Input: part model. Units: mm. Frame: model coordinates. Face numbers are marked on the shaded views. A direction names the side the tool comes from. Give positions to 0.01 mm unless a question says otherwise; leave off trailing zeros. Loops run counter-clockwise (first coordinate to the right, second up) from the corner with the lowest first, then second, coordinate; pieces in that order, holes last. Notation, with made-up numbers: (-38.5, 64) -> (-12.5, 64) arc R28 cw to (-12.5, 91) -> close; hole circle Ø1 at (65, -2.75). An arc over 180 degrees is marked (long way). Answer in a Markdown table with one row per item. Add a question column.
```python
from build123d import *

# Parameters (mm, degrees)
SKETCH1_W           = 57
SKETCH1_H           = 37
BOSS_EXTRUDE1_DEPTH = 44
SKETCH2_W           = 38.4
SKETCH2_H           = 36
CUT_EXTRUDE1_DEPTH  = 47
BOSS_EXTRUDE2_DEPTH = 20
BOSS_EXTRUDE3_DEPTH = 20
SKETCH7_W           = 53
SKETCH7_H           = 31
CUT_EXTRUDE4_DEPTH  = 8
SKETCH8_R           = 1.9
CUT_EXTRUDE5_DEPTH  = 40
SKETCH10_W          = 57
SKETCH10_H          = 77
BOSS_EXTRUDE4_DEPTH = 10
SKETCH12_W          = 38.4
SKETCH12_H          = 77
CUT_EXTRUDE6_DEPTH  = 8


with BuildPart() as part:
    # Sketch1 → Boss-Extrude1 (new body)
    with BuildSketch(Plane(origin=(0, 0, 0), x_dir=(1, 0, 0), z_dir=(0, 1, 0))):
        Rectangle(SKETCH1_W, SKETCH1_H)
    extrude(amount=BOSS_EXTRUDE1_DEPTH)

    # Sketch2 → Cut-Extrude1 (cut)
    with BuildSketch(Plane.XY.offset(18.5)):
        with Locations((0, 18)):
            Rectangle(SKETCH2_W, SKETCH2_H)
    extrude(amount=-CUT_EXTRUDE1_DEPTH, mode=Mode.SUBTRACT)

    # Sketch5 → Boss-Extrude2 (add)
    with BuildSketch(Plane(origin=(0, 0, -18.5), x_dir=(-1, 0, 0), z_dir=(0, 0, -1))):
        Polygon((-19.2, 36), (19.2, 36), (19.2, 0), (28.5, 0), (28.5, 44), (-28.5, 44), (-28.5, 0), (-19.2, 0), align=None)
    extrude(amount=BOSS_EXTRUDE2_DEPTH)

    # Sketch6 → Boss-Extrude3 (add)
    with BuildSketch(Plane.XY.offset(18.5)):
        Polygon((-28.5, 0), (-19.2, 0), (-19.2, 36), (19.2, 36), (19.2, 0), (28.5, 0), (28.5, 44), (-28.5, 44), align=None)
    extrude(amount=BOSS_EXTRUDE3_DEPTH)

    # Sketch7 → Cut-Extrude4 (cut)
    with BuildSketch(Plane(origin=(0, 44, 0), x_dir=(1, 0, 0), z_dir=(0, 1, 0))):
        with Locations((-2, 0)):
            Rectangle(SKETCH7_W, SKETCH7_H)
    extrude(amount=-CUT_EXTRUDE4_DEPTH, mode=Mode.SUBTRACT)

    # Sketch8 → Cut-Extrude5 (cut)
    with BuildSketch(Plane(origin=(0, 44, 0), x_dir=(1, 0, 0), z_dir=(0, 1, 0))):
        with Locations(Location((23.85, -27, 0), (0, 0, 270))):
            Circle(SKETCH8_R)
        with Locations(Location((-23.85, -27, 0), (0, 0, 270))):
            Circle(SKETCH8_R)
        with Locations(Location((-23.85, 27, 0), (0, 0, 270))):
            Circle(SKETCH8_R)
        with Locations(Location((23.85, 27, 0), (0, 0, 270))):
            Circle(SKETCH8_R)
    extrude(amount=-CUT_EXTRUDE5_DEPTH, mode=Mode.SUBTRACT)

    # Sketch10 → Boss-Extrude4 (add)
    with BuildSketch(Plane.XZ):
        Rectangle(SKETCH10_W, SKETCH10_H)
    extrude(amount=BOSS_EXTRUDE4_DEPTH)

    # Sketch12 → Cut-Extrude6 (cut)
    with BuildSketch(Plane(origin=(0, 44, 0), x_dir=(1, 0, 0), z_dir=(0, 1, 0))):
        Rectangle(SKETCH12_W, SKETCH12_H)
    extrude(amount=-CUT_EXTRUDE6_DEPTH, mode=Mode.SUBTRACT)


solid = part.part
```
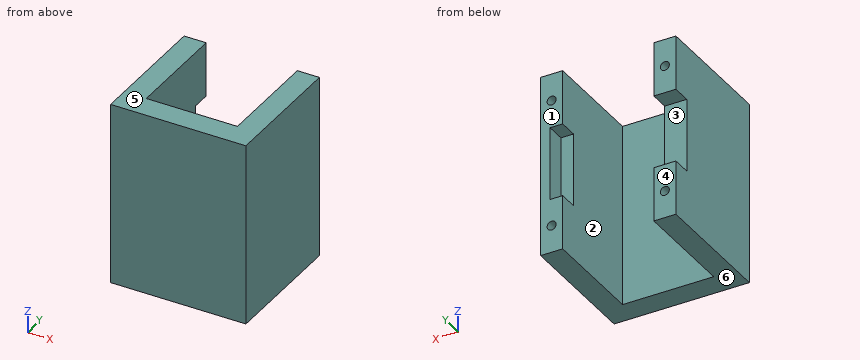
1) Section A-A on y = 6. Output: boundary loops of the cut face in (x, z), and give its area (3 significant figures).
2) Pin query (flat end, axial travel): pin 1 (4 mm diameter, centred on x = -7.5, z = -26.5, fed in from +Y); pin 2 (7.5 mm diameter, centred on x = -22, z = 4.5, fed in from +Y). Return the tip coordinate at first contact, or that it passes through.
3) Section C-C on x = -23.85. Output: boundary loops of the cut face in (y, z).
4) Section D-D on z = -27. Output: boundary loops of the cut face in (x, y).
5) Pull-direction query (Z, two-part tool) for the marked faces 3, 4, 5 and 6; classes: +Z half, -Z half, draft (parallel to the pull), parting line (faces both ways), or undercut.
6) Section B-B on z = 31. Output: boundary loops of the cut face in (x, y).
7) Material intervals for line 1 along X through (y, z) = (20, 27); line 2 along X through (y, z) = (14, -6); line 3 along Z through (x, y) = (-23, 23), sorted ascending.
8) Reachability of the marked faces 1 and 2 from +Z, -Z, +X, -X, +Y, -Y: full face, straight path, thin tool, end or side. Return the list, or none.
Working result:
| question | item | result |
|---|---|---|
| 1 | outline | (-28.5, -38.5) -> (-19.2, -38.5) -> (-19.2, 38.5) -> (-28.5, 38.5) -> close; (19.2, -38.5) -> (28.5, -38.5) -> (28.5, 38.5) -> (19.2, 38.5) -> close; hole circle Ø3.8 at (-23.85, -27); hole circle Ø3.8 at (-23.85, 27); hole circle Ø3.8 at (23.85, -27); hole circle Ø3.8 at (23.85, 27) |
| 1 | area | 1,390 mm2 |
| 2 | pin 1 | stops at y = 0 |
| 2 | pin 2 | stops at y = 36 |
| 3 | outline | (-10, -38.5) -> (44, -38.5) -> (44, -28.9) -> (4, -28.9) -> (4, -25.1) -> (44, -25.1) -> (44, -15.5) -> (36, -15.5) -> (36, 15.5) -> (44, 15.5) -> (44, 25.1) -> (4, 25.1) -> (4, 28.9) -> (44, 28.9) -> (44, 38.5) -> (-10, 38.5) -> close |
| 4 | outline | (-28.5, -10) -> (28.5, -10) -> (28.5, 44) -> (25.75, 44) -> (25.75, 4) -> (21.95, 4) -> (21.95, 44) -> (19.2, 44) -> (19.2, 0) -> (-19.2, 0) -> (-19.2, 44) -> (-21.95, 44) -> (-21.95, 4) -> (-25.75, 4) -> (-25.75, 44) -> (-28.5, 44) -> close |
| 5 | face 3 | undercut |
| 5 | face 4 | draft |
| 5 | face 5 | +Z half |
| 5 | face 6 | -Z half |
| 6 | outline | (-28.5, -10) -> (28.5, -10) -> (28.5, 44) -> (19.2, 44) -> (19.2, 0) -> (-19.2, 0) -> (-19.2, 44) -> (-28.5, 44) -> close |
| 7 | line 1 | x = -28.5 to -25.75, -21.95 to -19.2, 19.2 to 21.95, 25.75 to 28.5 |
| 7 | line 2 | x = -28.5 to -19.2, 19.2 to 28.5 |
| 7 | line 3 | z = -38.5 to -28.7, -25.3 to 25.3, 28.7 to 38.5 |
| 8 | face 1 | +Z, -Z, +X, -X, +Y |
| 8 | face 2 | +Z, -Z, +Y |
